Geometry: final body of the model. Coordinates: model frame, mm. A direction names the side the tool comes from. Give positions to 0.01 mm unless a question says otherwise; leave off trailing zeros. Write each loop counter-clockwise with the first axis right and the second up, starting at its lowest first coordinate (ties: lowest second). Pieces come first, ordered by that corner, then holes. Notation, with made-up numbers: M 40.25,32.25 L 70.25,32.25 A22 ccw 70.25,66.25 Z; hole C -11,69 d4. An arc over 180 degrees is marked long. Use one line per item in the form item = value. Start each with the question number.
Item 1: Section query D-D on y = 13.75. Return loops of the section in (x, z).
Item 2: Pull-direction query (X, two-part tool) for faces 1 (the flat face through (-0.2, 24, 35.4)), 2 (the cylindrical face through (-28, 4, -21)), 3 (the cylindrical face through (-8.67, 11.83, 39.05)); classes: released by +X, released by -X, zero draft, split by the parting line, or undercut.
Item 3: Contact query for flat-ended pins moving along their axis: P1, Ø1.5, axis at y = 10, z = -13.5, coming from the -X side; P2, Ø21, axis at x = 11.5, z = 7.5, coming from the -Y side; P3, Ø12, axis at x = 9, z = -0.5, coming from the +Y side. Output: stop coordinate, or through.
Item 4: Access query for faces 4 (the flat face through (0, 16, 0)), 5 (the flat face through (-0.2, 0, 35.4)), 6 (the flat face through (0, 8, 0)). Directions: +Z, -Z, +X, -X, +Y, -Y. A direction counts if a zero-diameter tool reaches every point of the face in a straight line with its end or side. Return the directions, or none.
Item 5: Section query C-C on y = 6. Return loops of the section in (x, z), then the cut area to 3 significant figures.
Item 6: Material intervals for line 1 along Z through (x, y) = (0, 20.5); line 2 along Y through (x, z) = (11, 16), sorted ascending. Write a range as from..to.
Item 7: Section query A-A on x = 0. Return loops of the section in (y, z), then the cut area to 3 significant figures.
Item 8: Section query B-B on z = 0. Return loops of the section in (x, y), then the cut area to 3 significant figures.
from build123d import *

# Parameters (mm, degrees)
ESQUISSE1_R             = 40
BOSS_EXTRU_1_DEPTH      = 24
ESQUISSE2_R             = 35
ENL_V_MAT_EXTRU_1_DEPTH = 8
ESQUISSE3_R             = 35
ENL_V_MAT_EXTRU_2_DEPTH = 8


with BuildPart() as part:
    # Esquisse1 → Boss.-Extru.1 (new body)
    with BuildSketch(Plane(origin=(0, 0, 0), x_dir=(1, 0, 0), z_dir=(0, 1, 0))):
        Circle(ESQUISSE1_R)
    extrude(amount=BOSS_EXTRU_1_DEPTH)

    # Esquisse2 → Enlèv. mat.-Extru.1 (cut)
    with BuildSketch(Plane(origin=(0, 24, 0), x_dir=(1, 0, 0), z_dir=(0, 1, 0))):
        Circle(ESQUISSE2_R)
    extrude(amount=-ENL_V_MAT_EXTRU_1_DEPTH, mode=Mode.SUBTRACT)

    # Esquisse3 → Enlèv. mat.-Extru.2 (cut)
    with BuildSketch(Plane.XZ):
        Circle(ESQUISSE3_R)
    extrude(amount=-ENL_V_MAT_EXTRU_2_DEPTH, mode=Mode.SUBTRACT)


solid = part.part
Answer sheet:
q1.outline = C 0,0 d80
q2.face_1 = zero draft
q2.face_2 = undercut
q2.face_3 = split by the parting line
q3.P1 = -37.91
q3.P2 = 8
q3.P3 = 16
q4.face_4 = +Y
q4.face_5 = +Z, -Z, +X, -X, -Y
q4.face_6 = -Y
q5.outline = C 0,0 d80; hole C 0,0 d70
q5.area = 1,180 mm2
q6.line_1 = -40..-35, 35..40
q6.line_2 = 8..16
q7.outline = M 0,-40 L 24,-40 L 24,-35 L 16,-35 L 16,35 L 24,35 L 24,40 L 0,40 L 0,35 L 8,35 L 8,-35 L 0,-35 Z
q7.area = 800 mm2
q8.outline = M -40,0 L -35,0 L -35,8 L 35,8 L 35,0 L 40,0 L 40,24 L 35,24 L 35,16 L -35,16 L -35,24 L -40,24 Z
q8.area = 800 mm2
